```python
from build123d import *

# Parameters (mm, degrees)
SKETCH_1_W      = 124
SKETCH_1_H      = 70
SKETCH_1_R      = 1.7
SKETCH_1_W_2    = 23
SKETCH_1_H_2    = 8
EXTRUDE_1_DEPTH = 2.5
FILLET_1_R      = 4
FILLET_2_R      = 4
FILLET_3_R      = 4
FILLET_4_R      = 4
FILLET_6_R      = 1
FILLET_8_R      = 1
FILLET_9_R      = 1


with BuildPart() as part:
    # 草图1 → 凸台-拉伸1 (new body)
    with BuildSketch(Plane(origin=(0, 0, 0), x_dir=(1, 0, 0), z_dir=(0, 1, 0))):
        with Locations((-5.316321244, -0.475281048)):
            Rectangle(SKETCH_1_W, SKETCH_1_H)
        with Locations((49.683678756, -30.975281048)):
            Circle(SKETCH_1_R, mode=Mode.SUBTRACT)
        with Locations((49.683678756, 30.024718952)):
            Circle(SKETCH_1_R, mode=Mode.SUBTRACT)
        with Locations((-60.316321244, 30.024718952)):
            Circle(SKETCH_1_R, mode=Mode.SUBTRACT)
        with Locations((-60.316321244, -30.975281048)):
            Circle(SKETCH_1_R, mode=Mode.SUBTRACT)
        with Locations((-42.316321244, -30.975281048)):
            Circle(SKETCH_1_R, mode=Mode.SUBTRACT)
        with Locations((-38.316321244, -25.475281048)):
            Circle(SKETCH_1_R, mode=Mode.SUBTRACT)
        with Locations((31.683678756, -30.975281048)):
            Circle(SKETCH_1_R, mode=Mode.SUBTRACT)
        with Locations((27.683678756, -25.475281048)):
            Circle(SKETCH_1_R, mode=Mode.SUBTRACT)
        with Locations((31.683678756, 30.024718952)):
            Circle(SKETCH_1_R, mode=Mode.SUBTRACT)
        with Locations((27.683678756, 24.524718952)):
            Circle(SKETCH_1_R, mode=Mode.SUBTRACT)
        with Locations((-42.316321244, 30.024718952)):
            Circle(SKETCH_1_R, mode=Mode.SUBTRACT)
        with Locations((-38.316321244, 24.524718952)):
            Circle(SKETCH_1_R, mode=Mode.SUBTRACT)
        with Locations((10.683678756, -25.675281048)):
            Rectangle(SKETCH_1_W_2, SKETCH_1_H_2, mode=Mode.SUBTRACT)
        with Locations((-21.316321244, -25.675281048)):
            Rectangle(SKETCH_1_W_2, SKETCH_1_H_2, mode=Mode.SUBTRACT)
        with Locations((-21.316321244, 24.724718952)):
            Rectangle(SKETCH_1_W_2, SKETCH_1_H_2, mode=Mode.SUBTRACT)
        with Locations((10.683678756, 24.724718952)):
            Rectangle(SKETCH_1_W_2, SKETCH_1_H_2, mode=Mode.SUBTRACT)
    extrude(amount=EXTRUDE_1_DEPTH)

    # 圆角1
    fillet_1_edges = [part.edges().sort_by_distance(p)[0] for p in [
        (-67.316321244, 1.25, 35.475281048),
    ]]
    fillet(fillet_1_edges, radius=FILLET_1_R)

    # 圆角2
    fillet_2_edges = [part.edges().sort_by_distance(p)[0] for p in [
        (-67.316321244, 1.25, -34.524718952),
    ]]
    fillet(fillet_2_edges, radius=FILLET_2_R)

    # 圆角3
    fillet_3_edges = [part.edges().sort_by_distance(p)[0] for p in [
        (56.683678756, 1.25, 35.475281048),
    ]]
    fillet(fillet_3_edges, radius=FILLET_3_R)

    # 圆角4
    fillet_4_edges = [part.edges().sort_by_distance(p)[0] for p in [
        (56.683678756, 1.25, -34.524718952),
    ]]
    fillet(fillet_4_edges, radius=FILLET_4_R)

    # 圆角6
    fillet_6_edges = [part.edges().sort_by_distance(p)[0] for p in [
        (-0.816321244, 1.25, -28.724718952),
        (-0.816321244, 1.25, -20.724718952),
        (22.183678756, 1.25, -20.724718952),
        (22.183678756, 1.25, -28.724718952),
    ]]
    fillet(fillet_6_edges, radius=FILLET_6_R)

    # 圆角8
    fillet_8_edges = [part.edges().sort_by_distance(p)[0] for p in [
        (-32.816321244, 1.25, -28.724718952),
        (-32.816321244, 1.25, -20.724718952),
        (-9.816321244, 1.25, -20.724718952),
        (-9.816321244, 1.25, -28.724718952),
    ]]
    fillet(fillet_8_edges, radius=FILLET_8_R)

    # 圆角9
    fillet_9_edges = [part.edges().sort_by_distance(p)[0] for p in [
        (-32.816321244, 1.25, 21.675281048),
        (-32.816321244, 1.25, 29.675281048),
        (-9.816321244, 1.25, 29.675281048),
        (-9.816321244, 1.25, 21.675281048),
        (-0.816321244, 1.25, 21.675281048),
        (-0.816321244, 1.25, 29.675281048),
        (22.183678756, 1.25, 29.675281048),
        (22.183678756, 1.25, 21.675281048),
    ]]
    fillet(fillet_9_edges, radius=FILLET_9_R)


solid = part.part
```
Geometry: final body of the model. Coordinates: model frame, mm. A direction names the side the tool comes from. Round coordinates to 2 decimals unless told otherwise and drop trailing zeros. Write each loop counter-clockwise with the first axis right and the second up, starting at its lowest first coordinate (ties: lowest second). Pieces come first, ordered by that corner, then holes. Notation, with made-up numbers: (-38.5, -3.5) -> (-7.5, -3.5) arc R22 ccw to (-7.5, 25.5) -> close; hole circle Ø10 at (65, -17). An arc over 180 degrees is marked (long way). Use CSV: the item, a comma, the result in double quotes. Start each with the question number.
Q1. Line query: L1, parallel to X at y = 2.05, z = 28.5; L2, parallel to Z at x = -15.5, y = 0.8; L3, parallel to X at y = 1.75, z = -29. Output: solid intervals per line, ascending.
Q2. Pull-direction query (Z, two-part tool) for faces 1 (the face through (-60.54, 1.23, 29.29)), 2 (the face through (-6, 0, 0)), 3 (the face through (-66.18, 1.27, 34.27)); classes: pulls with the +Z half, pulls with the -Z half, needs draft (parallel to the pull), parting line crosses it, or undercut.
Q3. Reachability of faces 4 (the face through (56.684, 1, 1)), 5 (the face through (-32.816, 1, -25)) from +Z, -Z, +X, -X, +Y, -Y: full face, straight path, thin tool, end or side. Return the list, or none.
Q4. Section C-C (y = 1.65). Give the number of separate pieces and of enclosed holes in the cut face, plus the area to 3 significant figures.
Q5. Section B-B (x = -38). Return loops of the section in (y, z), plus the area to 3 significant figures.
Q6. Section A-A (x = 5). Return loops of the section in (y, z), plus the area to 3 significant figures.
Result sheet:
1,L1,"-67.32 to -32.82, -9.82 to -0.82, 22.18 to 56.68"
1,L2,"-34.52 to -28.72, -20.72 to 21.68, 29.68 to 35.48"
1,L3,"-67.32 to -61.67, -58.96 to -43.67, -40.96 to 30.33, 33.04 to 48.33, 51.04 to 56.68"
2,face 1,"undercut"
2,face 2,"needs draft"
2,face 3,"pulls with the +Z half"
3,face 4,"+Z, -Z, +X, +Y, -Y"
3,face 5,"+Y, -Y"
4,separate pieces,"1"
4,enclosed holes,"16"
4,area,"7,820 mm²"
5,outline,"(0, -34.52) -> (2.5, -34.52) -> (2.5, -26.2) -> (0, -26.2) -> close; (0, -22.85) -> (2.5, -22.85) -> (2.5, 23.8) -> (0, 23.8) -> close; (0, 27.15) -> (2.5, 27.15) -> (2.5, 35.48) -> (0, 35.48) -> close"
5,area,"158 mm²"
6,outline,"(0, -34.52) -> (2.5, -34.52) -> (2.5, -28.72) -> (0, -28.72) -> close; (0, -20.72) -> (2.5, -20.72) -> (2.5, 21.68) -> (0, 21.68) -> close; (0, 29.68) -> (2.5, 29.68) -> (2.5, 35.48) -> (0, 35.48) -> close"
6,area,"135 mm²"
